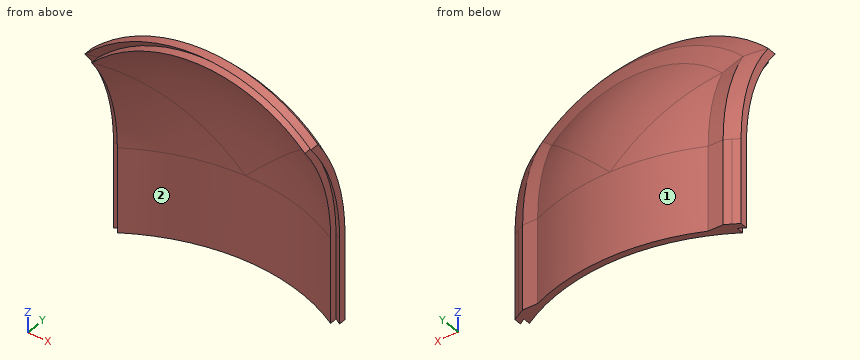
from build123d import *

# Parameters (mm, degrees)
EXTRUDE_1225_DEPTH     = 40
REVOLVE_1722_ANGLE     = 90
CUT_EXTRUDE_2087_DEPTH = 101
REVOLVE_2693_ANGLE     = 90


with BuildPart() as part:
    # 草图1 → Extrude 1225 (new body)
    with BuildSketch(Plane.XY):
        with BuildLine():
            Line((-50, 86.602540378), (-50, 83.120394609))
            ThreePointArc((-50, 83.120394609), (0, 97), (50, 83.120394609))
            Line((50, 83.120394609), (50, 86.602540378))
            ThreePointArc((50, 86.602540378), (45.070755856, 89.267166229), (40, 91.651513899))
            ThreePointArc((40, 91.651513899), (0, 100), (-40, 91.651513899))
            ThreePointArc((-40, 91.651513899), (-45.070755856, 89.267166229), (-50, 86.602540378))
        make_face()
        with BuildLine():
            ThreePointArc((40, 91.651513899), (45.070755856, 89.267166229), (50, 86.602540378))
            Line((50, 86.602540378), (50, 90.049986119))
            ThreePointArc((50, 90.049986119), (48.506610094, 90.863132112), (47, 91.651513899))
            Line((47, 91.651513899), (40, 91.651513899))
        make_face()
        with BuildLine():
            Line((50, 90.049986119), (50, 86.602540378))
            ThreePointArc((50, 86.602540378), (51.507887751, 85.714278271), (53, 84.799764151))
            Line((53, 84.799764151), (53, 88.317608663))
            ThreePointArc((53, 88.317608663), (51.507283785, 89.196410898), (50, 90.049986119))
        make_face()
        with BuildLine():
            Line((-50, 90.049986119), (-50, 86.602540378))
            ThreePointArc((-50, 86.602540378), (-45.070755856, 89.267166229), (-40, 91.651513899))
            Line((-40, 91.651513899), (-47, 91.651513899))
            ThreePointArc((-47, 91.651513899), (-48.506610094, 90.863132112), (-50, 90.049986119))
        make_face()
        with BuildLine():
            ThreePointArc((-53, 84.799764151), (-51.507887751, 85.714278271), (-50, 86.602540378))
            Line((-50, 86.602540378), (-50, 90.049986119))
            ThreePointArc((-50, 90.049986119), (-51.507283785, 89.196410898), (-53, 88.317608663))
            Line((-53, 88.317608663), (-53, 84.799764151))
        make_face()
    extrude(amount=-EXTRUDE_1225_DEPTH)

    # 草图5 → Revolve 1722 (revolve)
    with BuildSketch(Plane.XY):
        with BuildLine():
            Line((-50, 86.602540378), (-50, 83.120394609))
            ThreePointArc((-50, 83.120394609), (0, 97), (50, 83.120394609))
            Line((50, 83.120394609), (50, 86.602540378))
            ThreePointArc((50, 86.602540378), (51.507887751, 85.714278271), (53, 84.799764151))
            Line((53, 84.799764151), (53, 88.317608663))
            ThreePointArc((53, 88.317608663), (50.027779593, 90.034555971), (47, 91.651513899))
            Line((47, 91.651513899), (40, 91.651513899))
            ThreePointArc((40, 91.651513899), (0, 100), (-40, 91.651513899))
            Line((-40, 91.651513899), (-47, 91.651513899))
            ThreePointArc((-47, 91.651513899), (-50.027779593, 90.034555971), (-53, 88.317608663))
            Line((-53, 88.317608663), (-53, 84.799764151))
            ThreePointArc((-53, 84.799764151), (-51.507887751, 85.714278271), (-50, 86.602540378))
        make_face()
    revolve(axis=Axis((-50, 0, 0), (1, 0, 0)), revolution_arc=REVOLVE_1722_ANGLE)

    # 草图6 → Cut-Extrude 2087 (cut, through all)
    with BuildSketch(Plane(origin=(0, 0, 0), x_dir=(1, 0, 0), z_dir=(0, 1, 0))):
        with BuildLine():
            Line((0, 0), (-84.852813742, -84.852813742))
            ThreePointArc((-84.852813742, -84.852813742), (0, -120), (84.852813742, -84.852813742))
            Line((84.852813742, -84.852813742), (0, 0))
        make_face()
    extrude(amount=CUT_EXTRUDE_2087_DEPTH, mode=Mode.SUBTRACT)

    # 草图7 → Revolve 2693 (revolve)
    with BuildSketch(Plane(origin=(0, 0, 0), x_dir=(0.707106781, 0, -0.707106781), z_dir=(0.707106781, 0, 0.707106781))):
        with BuildLine():
            Line((-74.953318806, 70.647009845), (-74.953318806, 66.196676654))
            ThreePointArc((-74.953318806, 66.196676654), (-72.866961322, 68.486538441), (-70.710678119, 70.710678119))
            Line((-70.710678119, 70.710678119), (-70.710678119, 66.400301204))
            ThreePointArc((-70.710678119, 66.400301204), (-38.52382888, 89.021989466), (0, 97))
            Line((0, 97), (0, 100))
            ThreePointArc((0, 100), (-29.612402374, 95.514949749), (-56.568542495, 82.462112512))
            add(Edge.make_bspline(
                [(-56.568542495, 82.462112512), (-61.63437241, 80.724547186), (-66.468037432, 78.682907928)],
                knots=[5.164022421, 5.164022421, 5.164022421, 5.250846104, 5.250846104, 5.250846104], degree=2, weights=[1, 0.999057854, 1]))
            ThreePointArc((-66.468037432, 78.682907928), (-70.824740836, 74.785400216), (-74.953318806, 70.647009845))
        make_face()
    revolve(axis=Axis((0, 0, 0), (0, 1, 0)), revolution_arc=REVOLVE_2693_ANGLE)


solid = part.part
Geometry: final body of the model. Coordinates: model frame, mm. Face numbers are marked on the shaded views. Round coordinates to 2 decimals unless told otherwise and drop trailing zeros. Loops run counter-clockwise (first coordinate to the right, second up) from the corner with the lowest first, then second, coordinate; pieces in that order, holes last. Notation, with made-up numbers: (81, 58) - (118, 58) arc R22 ccw to (118, 94) - close; hole circle Ø8 at (16.25, -40). An arc over 180 degrees is marked (long way). Write each question's results on one line, items separated by ' | '. Start each with the question number.
1) Line query: probe 1 along X at (y, z) = (89, -8.5); probe 2 along X at (y, z) = (74, 55); probe 3 along Z at (x, y) = (22.5, 69.5). Output: solid intervals per line, ascending. Write a range as [from, to].
2) Cut plane B-B on y = 94. Return loops of the section in (x, z).
3) Mould query, pull axis X, two halves, no side actions, for the marked faces 1 and 2. Classes: released by +X, released by -X, zero draft, split by the parting line, or undercut.
4) First-contact query: P1, Ø12, axis at x = -25, z = -18.5, coming from the -Y side; P2, Ø4, axis at x = -21, z = 56.5, coming from the -Y side; P3, Ø3.5, axis at x = -42.5, z = -27, coming from the +Y side. Flat tips, straight axial feed; report the tip coordinate or a pass-through.
5) Cut plane A-A on z = -11. Return loops of the section in (x, y), then the cut area to 3 significant figures.
Verdict:
1) probe 1: x = [-51.85, -38.57], [38.57, 51.85] | probe 2: x = [-45.91, -30.13], [30.13, 45.91] | probe 3: z = [63.82, 67.04], [68.29, 71.5]
2) outline: (-34.12, -40) - (-23.94, -40) - (-23.94, 0) arc R23.94 cw to (23.94, 0) - (23.94, -40) - (34.12, -40) - (34.12, 0) arc R34.12 ccw to (-34.12, 0) - close
3) face 1: split by the parting line | face 2: undercut
4) P1: stops at y = 91.91 | P2: stops at y = 74.37 | P3: stops at y = 91.65
5) outline: (-53, 84.8) arc R100 cw to (-50, 86.6) - (-50, 83.12) arc R97 cw to (50, 83.12) - (50, 86.6) arc R100 cw to (53, 84.8) - (53, 88.32) arc R103 ccw to (47, 91.65) - (40, 91.65) arc R100 ccw to (-40, 91.65) - (-47, 91.65) arc R103 ccw to (-53, 88.32) - close | area: 379 mm2
